CAD build for the part. Positions are in the model's coordinates, mm. Give positions to 0.01 mm unless a question says otherwise; leave off trailing zeros. Write each loop counter-clockwise with the first axis right and the second up, starting at its lowest first coordinate (ties: lowest second). Pieces come first, ordered by that corner, then holes. Notation, with made-up numbers: (66, 28.25) - (85, 28.25) arc R25 ccw to (85, 58.25) - close; hole circle Ø1 at (-22.75, 16). An arc over 180 degrees is marked (long way). Answer as a JSON object with one key per item and string values.
from build123d import *

# Parameters (mm, degrees)
SKETCH_1_W          = 60
SKETCH_1_H          = 80
EXTRUDE_1_DEPTH     = 2
SKETCH_2_R          = 1.4
CUT_EXTRUDE_1_DEPTH = 50
SKETCH_3_R          = 2
CUT_EXTRUDE_2_DEPTH = 50
SKETCH_5_W          = 60
SKETCH_5_H          = 40
EXTRUDE_2_DEPTH     = 2
SKETCH_6_R          = 20
CUT_EXTRUDE_4_DEPTH = 50
SKETCH_4_R          = 1.65
CUT_EXTRUDE_3_DEPTH = 50
SKETCH_7_R          = 1.6
CUT_EXTRUDE_5_DEPTH = 10
SKETCH_11_W         = 60
SKETCH_11_H         = 35
EXTRUDE_3_DEPTH     = 2
FILLET_1_R          = 10
SKETCH_13_R         = 1.6
CUT_EXTRUDE_6_DEPTH = 10
SKETCH_17_R         = 1.6
CUT_EXTRUDE_7_DEPTH = 10


with BuildPart() as part:
    # 草图1 → 凸台-拉伸1 (new body)
    with BuildSketch(Plane(origin=(0, 0, 0), x_dir=(1, 0, 0), z_dir=(0, 1, 0))):
        Rectangle(SKETCH_1_W, SKETCH_1_H)
    extrude(amount=EXTRUDE_1_DEPTH)

    # 草图2 → 切除-拉伸1 (cut)
    with BuildSketch(Plane(origin=(0, 2, 0), x_dir=(1, 0, 0), z_dir=(0, 1, 0))):
        with Locations(Location((0, -10.50070918, 0), (0, 0, 270))):
            Circle(SKETCH_2_R)
        with Locations(Location((9.49929082, -20, 0), (0, 0, 270))):
            Circle(SKETCH_2_R)
        with Locations(Location((0, -29.49929082, 0), (0, 0, 270))):
            Circle(SKETCH_2_R)
        with Locations(Location((-9.49929082, -20, 0), (0, 0, 270))):
            Circle(SKETCH_2_R)
    extrude(amount=-CUT_EXTRUDE_1_DEPTH, mode=Mode.SUBTRACT)

    # 草图3 → 切除-拉伸2 (cut)
    with BuildSketch(Plane(origin=(0, 2, 0), x_dir=(1, 0, 0), z_dir=(0, 1, 0))):
        with Locations(Location((0, -20, 0), (0, 0, 270))):
            Circle(SKETCH_3_R)
    extrude(amount=-CUT_EXTRUDE_2_DEPTH, mode=Mode.SUBTRACT)

    # 草图5 → 凸台-拉伸2 (add)
    with BuildSketch(Plane(origin=(0, 2, 0), x_dir=(1, 0, 0), z_dir=(0, 1, 0))):
        with Locations((0, 60)):
            Rectangle(SKETCH_5_W, SKETCH_5_H)
    extrude(amount=-EXTRUDE_2_DEPTH)

    # 草图6 → 切除-拉伸4 (cut)
    with BuildSketch(Plane(origin=(0, 2, 0), x_dir=(1, 0, 0), z_dir=(0, 1, 0))):
        with Locations(Location((0, 32, 0), (0, 0, 270))):
            Circle(SKETCH_6_R)
    cut_extrude_4 = extrude(amount=-CUT_EXTRUDE_4_DEPTH, mode=Mode.SUBTRACT)

    # 草图4 → 切除-拉伸3 (cut)
    with BuildSketch(Plane(origin=(0, 2, 0), x_dir=(1, 0, 0), z_dir=(0, 1, 0))):
        with Locations(Location((-8, 73.5, 0), (0, 0, 270))):
            Circle(SKETCH_4_R)
        with Locations(Location((8, 73.5, 0), (0, 0, 270))):
            Circle(SKETCH_4_R)
        with Locations(Location((8, 60.5, 0), (0, 0, 270))):
            Circle(SKETCH_4_R)
        with Locations(Location((-8, 60.5, 0), (0, 0, 270))):
            Circle(SKETCH_4_R)
    cut_extrude_3 = extrude(amount=-CUT_EXTRUDE_3_DEPTH, mode=Mode.SUBTRACT)

    # 草图7 → 切除-拉伸5 (cut)
    with BuildSketch(Plane(origin=(0, 2, 0), x_dir=(1, 0, 0), z_dir=(0, 1, 0))):
        with Locations(Location((-25.5, 20, 0), (0, 0, 270))):
            Circle(SKETCH_7_R)
        with Locations(Location((-25.5, 5, 0), (0, 0, 270))):
            Circle(SKETCH_7_R)
        with Locations(Location((-25.5, -10, 0), (0, 0, 270))):
            Circle(SKETCH_7_R)
        with Locations(Location((-25.5, -25, 0), (0, 0, 270))):
            Circle(SKETCH_7_R)
        with Locations(Location((-25.5, 35, 0), (0, 0, 270))):
            Circle(SKETCH_7_R)
        with Locations(Location((-25.5, 50, 0), (0, 0, 270))):
            Circle(SKETCH_7_R)
        with Locations(Location((-25.5, 65, 0), (0, 0, 270))):
            Circle(SKETCH_7_R)
        with Locations(Location((25.5, 65, 0), (0, 0, 270))):
            Circle(SKETCH_7_R)
        with Locations(Location((25.5, 50, 0), (0, 0, 270))):
            Circle(SKETCH_7_R)
        with Locations(Location((25.5, 35, 0), (0, 0, 270))):
            Circle(SKETCH_7_R)
        with Locations(Location((25.5, -25, 0), (0, 0, 270))):
            Circle(SKETCH_7_R)
        with Locations(Location((25.5, -10, 0), (0, 0, 270))):
            Circle(SKETCH_7_R)
        with Locations(Location((25.5, 5, 0), (0, 0, 270))):
            Circle(SKETCH_7_R)
        with Locations(Location((25.5, 20, 0), (0, 0, 270))):
            Circle(SKETCH_7_R)
    extrude(amount=-CUT_EXTRUDE_5_DEPTH, mode=Mode.SUBTRACT)

    # 草图11 → 凸台-拉伸3 (add)
    with BuildSketch(Plane(origin=(0, 2, 0), x_dir=(1, 0, 0), z_dir=(0, 1, 0))):
        with Locations((0, -57.5)):
            Rectangle(SKETCH_11_W, SKETCH_11_H)
    extrude(amount=-EXTRUDE_3_DEPTH)

    # 镜向2: 切除-拉伸4, 切除-拉伸3 across plane
    add(cut_extrude_4.mirror(Plane.XY.offset(-6)), mode=Mode.SUBTRACT)
    add(cut_extrude_3.mirror(Plane.XY.offset(-6)), mode=Mode.SUBTRACT)

    # 圆角1
    fillet_1_edges = [part.edges().sort_by_distance(p)[0] for p in [
        (-30, 1, 75),
        (30, 1, 75),
        (-30, 1, -80),
        (30, 1, -80),
    ]]
    fillet(fillet_1_edges, radius=FILLET_1_R)

    # 草图13 → 切除-拉伸6 (cut)
    with BuildSketch(Plane(origin=(0, 0, 0), x_dir=(-1, 0, 0), z_dir=(0, -1, 0))):
        with Locations(Location((-25.5, -60, 0), (0, 0, 90))):
            Circle(SKETCH_13_R)
        with Locations(Location((25.5, -60, 0), (0, 0, 270))):
            Circle(SKETCH_13_R)
    extrude(amount=-CUT_EXTRUDE_6_DEPTH, mode=Mode.SUBTRACT)

    # 草图17 → 切除-拉伸7 (cut)
    with BuildSketch(Plane(origin=(0, 2, 0), x_dir=(1, 0, 0), z_dir=(0, 1, 0))):
        with Locations(Location((-25.5, -40, 0), (0, 0, 270))):
            Circle(SKETCH_17_R)
        with Locations(Location((25.5, -40, 0), (0, 0, 270))):
            Circle(SKETCH_17_R)
    extrude(amount=-CUT_EXTRUDE_7_DEPTH, mode=Mode.SUBTRACT)


solid = part.part
Item 1: Cut at D-D (x = 8). Give the cut face in (y, z).
Entries:
{"outline": "(0, -80) - (2, -80) - (2, -75.15) - (0, -75.15) - close; (0, -71.85) - (2, -71.85) - (2, -62.15) - (0, -62.15) - close; (0, -58.85) - (2, -58.85) - (2, -50.33) - (0, -50.33) - close; (0, -13.67) - (2, -13.67) - (2, 1.67) - (0, 1.67) - close; (0, 38.33) - (2, 38.33) - (2, 46.85) - (0, 46.85) - close; (0, 50.15) - (2, 50.15) - (2, 59.85) - (0, 59.85) - close; (0, 63.15) - (2, 63.15) - (2, 75) - (0, 75) - close"}
Item 2: Probe line 1 (X direction, y = 1.75, z = -5); line 2 (X direction, y = 0.75, z = 48.5); line 3 (X direction, y = 0.8, z = -33). List the from-to ranges inside material, lowest first. Write a range as from..to.
Entries:
{"line 1": "-30..-27.1, -23.9..23.9, 27.1..30", "line 2": "-30..-9.65, -6.35..6.35, 9.65..30", "line 3": "-30..-19.97, 19.97..30"}
Item 3: Cut at C-C (x = 0). Give the cut face in (y, z).
Entries:
{"outline": "(0, -80) - (2, -80) - (2, -52) - (0, -52) - close; (0, -12) - (2, -12) - (2, 0) - (0, 0) - close; (0, 40) - (2, 40) - (2, 75) - (0, 75) - close"}
Item 4: Cut at A-A (z = -5). Give the cut face in (x, y).
Entries:
{"outline": "(-30, 0) - (-27.1, 0) - (-27.1, 2) - (-30, 2) - close; (-23.9, 0) - (23.9, 0) - (23.9, 2) - (-23.9, 2) - close; (27.1, 0) - (30, 0) - (30, 2) - (27.1, 2) - close"}
Item 5: Cut at B-B (z = -32). Give the cut face in (x, y).
Entries:
{"outline": "(-30, 0) - (-20, 0) - (-20, 2) - (-30, 2) - close; (20, 0) - (30, 0) - (30, 2) - (20, 2) - close"}
Item 6: Mould opens along X. For faces 1 (the cylindrical face through (-27.15, 0.99, -76.99)), 2 (the flat face through (0, 2, -4)), 3 (the cylindrical face through (8.07, 1.01, 50.15)) say: +X half, -X half, draft (parallel to the pull), parting line (faces both ways), or undercut.
Entries:
{"face 1": "-X half", "face 2": "draft", "face 3": "undercut"}
